Check sheet for the drawn part. Datum: minimum x, y, z corner. Units: mm. A direction names the side the tool comes from. Give positions to 0.01 mm unless a question says otherwise; leave off trailing zeros. Write each loop counter-clockwise with the first axis right and the second up, starting at its lowest first coordinate (ties: lowest second). Pieces come first, ordered by that corner, then holes. Notation, with made-up numbers: (52, 44) - (72, 44) arc R18 cw to (72, 66) - close; hole circle Ø3 at (-8, 89). An arc over 180 degrees is marked (long way). Answer as a JSON object with one key per item and string values. Group by question number.
Item 1: Tool access check on the marked faces 1 and 2. Record the directions out of +Z, -Z, +X, -X, +Y, -Y that give a thin tool (end or side, any length) a straight path to the whole face; none if there is none.
Item 2: Go/stop test with flat-tipped pins: pin 1 (6 mm diameter, centred on x = 125.75, z = 12.7, fed in from +Y); pin 2 (6 mm diameter, centred on x = 146, z = 61, fed in from -Y) (3 decimals). Record where each tip stops, or that it passes through.
Item 3: Sectioned sample at B-B, the plane x = 25.4. Record the boundary of the cut face in (y, z) (3 decimals).
Item 4: Scan lines: line 1 along X through (y, z) = (50, 12); line 2 along Z through (x, y) = (122.5, 11) (3 decimals); line 3 along Y through (x, z) = (128, 33) (3 decimals). Record each from-to range of solid material in increasing order. Write a range as [from, to].
Item 5: Sectioned sample at D-D, the plane z = 49.5. Record the boundary of the cut face in (x, y) (3 decimals).
Item 6: Sectioned sample at C-C, the plane x = 68. Record the boundary of the cut face in (y, z) (3 decimals), and give its area (3 significant figures).
Item 7: Sectioned sample at A-A, the plane z = 12.7. Record the boundary of the cut face in (x, y) (3 decimals), and give its area (3 significant figures).
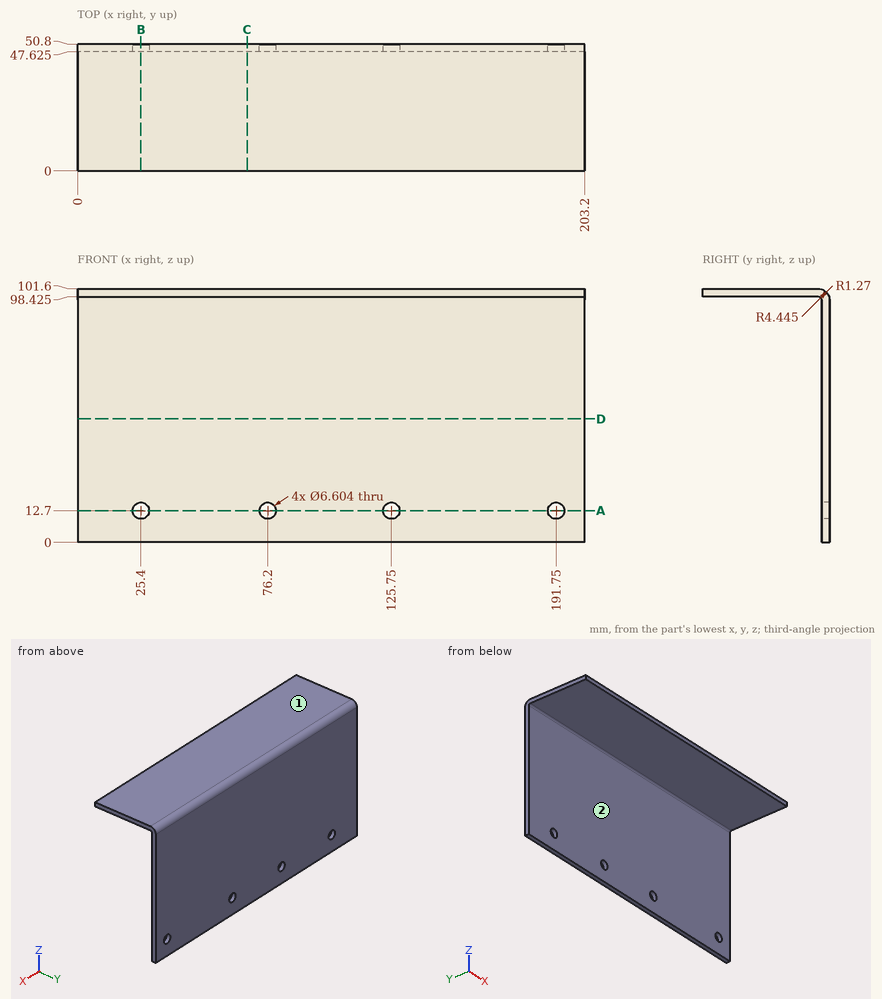
Geometry check:
{
 "1": {"face 1": "+Z, +X, -X, +Y, -Y", "face 2": "-Z, +X, -X, -Y"},
 "2": {"pin 1": "through", "pin 2": "y = 47.625"},
 "3": {"outline": "(0, 98.425) - (46.355, 98.425) arc R1.27 cw to (47.625, 97.155) - (47.625, 16.002) - (50.8, 16.002) - (50.8, 97.155) arc R4.445 ccw to (46.355, 101.6) - (0, 101.6) - close; (47.625, 0) - (50.8, 0) - (50.8, 9.398) - (47.625, 9.398) - close"},
 "4": {"line 1": "[0, 22.17], [28.63, 72.97], [79.43, 122.52], [128.98, 188.52], [194.98, 203.2]", "line 2": "[98.425, 101.6]", "line 3": "[47.625, 50.8]"},
 "5": {"outline": "(0, 47.625) - (203.2, 47.625) - (203.2, 50.8) - (0, 50.8) - close"},
 "6": {"outline": "(0, 98.425) - (46.355, 98.425) arc R1.27 cw to (47.625, 97.155) - (47.625, 0) - (50.8, 0) - (50.8, 97.155) arc R4.445 ccw to (46.355, 101.6) - (0, 101.6) - close", "area": "470 mm^2"},
 "7": {"outline": "(0, 47.625) - (22.098, 47.625) - (22.098, 50.8) - (0, 50.8) - close; (28.702, 47.625) - (72.898, 47.625) - (72.898, 50.8) - (28.702, 50.8) - close; (79.502, 47.625) - (122.448, 47.625) - (122.448, 50.8) - (79.502, 50.8) - close; (129.052, 47.625) - (188.448, 47.625) - (188.448, 50.8) - (129.052, 50.8) - close; (195.052, 47.625) - (203.2, 47.625) - (203.2, 50.8) - (195.052, 50.8) - close", "area": "561 mm^2"}
}
